The listing builds one solid part. Answer for the finished solid, in the listing's coordinates (mm). A direction names the side the tool comes from. Coordinates: 2 decimals unless noted, no trailing zeros. Order: outer loops, then holes, each group sorted by start corner. A loop starts at its lowest first (then second) coordinate and runs counter-clockwise, first axis right, second up. Notation, with made-up numbers: M -18,80.5 L -8,80.5 A38 cw -8,119.5 Z; hole C 43,-33.5 d1. An arc over 180 degrees is marked long. One line per item, written item: value. Start each with the question number.
Q1. The part is cut by section C-C on z = 25. Give the vertices of the cut face in (x, y), then the cut area to 3 significant figures.
Q2. The part is cut by section B-B on z = -7.5. Give the vertices of the cut face in (x, y).
Q3. For faces 1 (the flat face through (22.4, 0, -36.2)), 2 (the flat face through (0, 0, 0)), determine the directions among +Z, -Z, +X, -X, +Y, -Y from which every point of the face is accessible in a straight line to the end or side of a thin tool.
Q4. Determine the mould class of faces 3 (the cylindrical face through (25.77, -0.02, -30)), 4 (the cylindrical face through (1.43, -0.02, 11.95)), 5 (the cylindrical face through (18.275, -0.021, -42.295)) for opening direction X: pulls with the +X half, pulls with the -X half, needs draft (parallel to the pull), parting line crosses it, or undercut.
Q5. Straight lines are drawn through the part: line 1 along Z through (x, y) = (1, 0.6); line 2 along X through (y, z) = (0.8, -7.5); line 3 along X through (y, z) = (0, -6.5). For each, find the intervals that lie inside material, in ascending order. Write a range as [from, to].
Q6. The part is cut by section D-D on y = 0.95. Give the number of separate pieces and of enclosed holes in the cut face, then the cut area to 3 significant figures.
Q7. The part is cut by section A-A on x = -25. Give the vertices of the cut face in (y, z), then the cut area to 3 significant figures.
Q8. Each of these flat-tipped pins is pushed along its axis until it touches: pin 1 Ø4.5 at (x, z) = (-5, -7.5) entering from -Y; pin 2 Ø1.5 at (y, z) = (0, 6.5) entering from -X (3 decimals); pin 3 Ø0.9 at (x, y) = (-18.5, -0.5) entering from +Z. Where does it stop, or does it pass through?
```python
from build123d import *

# Parameters (mm, degrees)
SKETCH_4_R                   = 1.6
EXTRUDE_1_DEPTH              = 1.5
CUT_EXTRUDE_2_DEPTH          = 3
FILLET_2_R                   = 1.75
HOLE_WIZARD_M3_1_D           = 3.4
HOLE_WIZARD_M3_1_DEPTH       = 5.978536948
HOLE_WIZARD_M3_1_CSINK_D     = 6.3
HOLE_WIZARD_M3_1_CSINK_ANGLE = 90
HOLE_WIZARD_M3_1_TIP         = 1.021463052


with BuildPart() as part:
    # ｽｹｯﾁ4 → ﾎﾞｽ - 押し出し1 (new, symmetric)
    with BuildSketch(Plane(origin=(0, 0, 0), x_dir=(1, 0, 0), z_dir=(0, 1, 0))):
        Polygon((-30, 0), (-30, 15), (18.480762114, 42.990381057), (25.980762114, 30), (0, -30), (-15, -30), align=None)
        with Locations(Location((0.580127019, 23.995190528, 0), (0, 0, 270))):
            Circle(SKETCH_4_R, mode=Mode.SUBTRACT)
        with Locations(Location((-5, 7.5, 0), (0, 0, 270))):
            Circle(SKETCH_4_R, mode=Mode.SUBTRACT)
        with Locations(Location((-7.5, -5, 0), (0, 0, 270))):
            Circle(SKETCH_4_R, mode=Mode.SUBTRACT)
        with Locations(Location((-7.5, -25, 0), (0, 0, 270))):
            Circle(SKETCH_4_R, mode=Mode.SUBTRACT)
        with Locations(Location((-25, 7.5, 0), (0, 0, 270))):
            Circle(SKETCH_4_R, mode=Mode.SUBTRACT)
        with Locations(Location((17.900635095, 33.995190528, 0), (0, 0, 270))):
            Circle(SKETCH_4_R, mode=Mode.SUBTRACT)
    extrude(amount=EXTRUDE_1_DEPTH, both=True)

    # ｽｹｯﾁ5 → ｶｯﾄ - 押し出し2 (cut)
    with BuildSketch(Plane(origin=(0, 1.5, 0), x_dir=(1, 0, 0), z_dir=(0, 1, 0))):
        Polygon((12.665448219, 10.574351407), (19.442413698, 26.225082782), (6.92820323, 19), (4.714101615, 15.165063509), align=None)
        Polygon((4.714101615, 15.165063509), (6.92820323, 19), (2.5, 16.443375673), align=None)
        Polygon((2.214101615, 10.834936491), (0, 12.113248654), (0, 7), align=None)
        Polygon((0, 0), (0, -18.675248347), (10.665448219, 5.955549254), (2.214101615, 10.834936491), (0, 7), align=None)
        Polygon((-15, 0), (-24.968847051, 0), (-15, -19.937694101), align=None)
    extrude(amount=-CUT_EXTRUDE_2_DEPTH, mode=Mode.SUBTRACT)

    # ﾌｨﾚｯﾄ2
    fillet_2_edges = [part.edges().sort_by_distance(p)[0] for p in [
        (-30, 0, 0),
        (-30, 0, -15),
        (18.480762114, 0, -42.990381057),
        (25.980762114, 0, -30),
        (0, 0, 30),
        (-15, 0, 30),
        (-24.968847051, 0, 0),
        (-15, 0, 0),
        (-15, 0, 19.937694101),
        (0, 0, 18.675248347),
        (0, 0, -12.113248654),
        (10.665448219, 0, -5.955549254),
        (2.5, 0, -16.443375673),
        (19.442413698, 0, -26.225082782),
        (12.665448219, 0, -10.574351407),
    ]]
    fillet(fillet_2_edges, radius=FILLET_2_R)

    # M3 丸皿ねじ用皿穴1
    with Locations(Plane(origin=(-7.5, -1.5, 25), x_dir=(0, 0, -1), z_dir=(0, -1, 0))):
        with Locations((0, 0), (20, 0), (32.5, -17.5), (32.5, 2.5), (48.995190528, 8.080127019), (58.995190528, 25.400635095)):
            CounterSinkHole(HOLE_WIZARD_M3_1_D / 2, HOLE_WIZARD_M3_1_CSINK_D / 2, depth=HOLE_WIZARD_M3_1_DEPTH, counter_sink_angle=HOLE_WIZARD_M3_1_CSINK_ANGLE)
            with Locations((0, 0, -(HOLE_WIZARD_M3_1_DEPTH + HOLE_WIZARD_M3_1_TIP / 2))):  # 118° drill point
                Cone(0, HOLE_WIZARD_M3_1_D / 2, HOLE_WIZARD_M3_1_TIP, mode=Mode.SUBTRACT)


solid = part.part
```
Output:
1. outline: M -17.5,-1.5 L -10.65,-1.5 L -9.2,-0.05 L -9.2,1.5 L -17.5,1.5 Z; M -5.8,-0.05 L -4.35,-1.5 L 2.17,-1.5 L 2.17,1.5 L -5.8,1.5 Z
1. area: 46.7 mm^2
2. outline: M -30,-1.5 L -28.15,-1.5 L -26.7,-0.05 L -26.7,1.5 L -30,1.5 Z; M -23.3,-0.05 L -21.85,-1.5 L -8.15,-1.5 L -6.7,-0.05 L -6.7,1.5 L -23.3,1.5 Z; M -3.3,-0.05 L -1.85,-1.5 L 0,-1.5 L 0,1.5 L -3.3,1.5 Z; M 7.99,-1.5 L 16.24,-1.5 L 16.24,1.5 L 7.99,1.5 Z
3. face 1: -Z, +X, +Y, -Y
3. face 2: +Y, -Y
4. face 3: pulls with the +X half
4. face 4: undercut
4. face 5: parting line crosses it
5. line 1: z = [-32.9, -25.64], [-22.35, -10.66], [11.81, 27.69]
5. line 2: x = [-30, -26.7], [-23.3, -6.7], [-3.3, 0], [7.99, 16.24]
5. line 3: x = [-30, -26.37], [-23.63, -6.37], [-3.63, 0], [9.63, 15.8]
6. separate pieces: 1
6. enclosed holes: 9
6. area: 1,970 mm^2
7. outline: M -1.5,-17.89 L 1.5,-17.89 L 1.5,-9.2 L -0.05,-9.2 L -1.5,-10.65 Z; M -1.5,-4.35 L -0.05,-5.8 L 1.5,-5.8 L 1.5,10 L -1.5,10 Z
7. area: 71.4 mm^2
8. pin 1: stops at y = -0.6
8. pin 2: stops at x = -27.125
8. pin 3: stops at z = 23.9
